Model file for the job. Use its own axes, mm. A direction names the side the tool comes from. Round coordinates to 2 decimals unless told otherwise and drop trailing zeros. Order: outer loops, then holes, each group sorted by start corner. A loop starts at its lowest first (then second) coordinate and runs counter-clockwise, first axis right, second up. Notation, with made-up numbers: (89, 50.25) - (141, 50.25) arc R23 cw to (141, 80.25) - close; hole circle Ø9 at (88, 68.5). An arc over 180 degrees is marked (long way). Put each result on its own line as item: value. Start each with the question number.
Item 1: Pin check, flat tips, straight feed: pin 1 Ø8 at (x, z) = (53, -35) entering from +Y; pin 2 Ø8 at (y, z) = (49, -28.5) entering from -X; pin 3 Ø3 at (y, z) = (53, -13.5) entering from -X. Stop position of each tip, or through.
Item 2: Saw through at B-B on x = 50. List the corners of the cut face in (y, z).
Item 3: Saw through at C-C on z = -88. List the corners of the cut face in (x, y).
Item 4: Saw through at A-A on z = -47. List the corners of the cut face in (x, y).
Item 5: Saw through at D-D on x = 16.5. List the corners of the cut face in (y, z), plus the area to 3 significant figures.
Item 6: Which spindle directions (+Z, -Z, +X, -X, +Y, -Y) get a long thin tool onto all of the face, cutting with end or side? Do faces 1 (the face through (49.349, 57.395, -45.043)), 2 (the face through (49, 25, 0)). Say none if no direction does.
Item 7: Probe probe 1 along Y at (x, z) = (32.5, -81). List the from-to ranges inside material, lowest first.
Autodesk Inventor part; units mm, degrees
ref_plane "YZ Plane" through (0, 0, 0) normal (1, 0, 0) x (0, 1, 0)
ref_plane "XZ Plane" through (0, 0, 0) normal (0, 1, 0) x (-1, 0, 0)
ref_plane "XY Plane" through (0, 0, 0) normal (0, 0, 1) x (1, 0, 0)
sketch "Sketch1" plane through (0, 0, 0) normal (0, 1, 0) x (-1, 0, 0)
  point P0 (0, 0)
sketch "Sketch2" plane through (0, 0, 0) normal (0, 1, 0) x (-1, 0, 0)
  line L0 (0, 0) -> (-100, 0)
  line L1 (-100, 0) -> (-100, -100)
  line L2 (-100, -100) -> (0, -100)
  line L3 (0, -100) -> (0, 0)
  dimension "d0" = 100
  dimension "d1" = 100
extrude "Extrusion1" add sketch "Sketch2" along normal blind 50
sketch "Sketch3" plane through (0, 50, 0) normal (0, 1, 0) x (1, 0, 0)
  circle A0 centre (50, 50) radius 5
  point P0 (0, 0)
  dimension "d4" = 10
extrude "Extrusion2" add sketch "Sketch3" along normal blind 15
sketch "Sketch4" plane through (50, 65, -50) normal (0, 1, 0) x (1, 0, 0)
  point P0 (-50, -50)
properties part number "Base"
Results found:
1. pin 1: stops at y = 50
1. pin 2: stops at x = 0
1. pin 3: passes through
2. outline: (0, -100) - (50, -100) - (50, -55) - (65, -55) - (65, -45) - (50, -45) - (50, 0) - (0, 0) - close
3. outline: (0, 0) - (100, 0) - (100, 50) - (0, 50) - close
4. outline: (0, 0) - (100, 0) - (100, 50) - (54, 50) - (54, 65) - (46, 65) - (46, 50) - (0, 50) - close
5. outline: (0, -100) - (50, -100) - (50, 0) - (0, 0) - close
5. area: 5,000 mm²
6. face 1: +Y
6. face 2: +Z, +X, -X, +Y, -Y
7. probe 1: y = 0 to 50
